Design review of the part built by this model. Coordinates are the model's own, in mm. Face numbers are marked on the shaded views. A direction names the side the tool comes from. Give positions to 0.01 mm unless a question says otherwise; leave off trailing zeros. Order: outer loops, then holes, each group sorted by start corner. A loop starts at its lowest first (then second) coordinate and runs counter-clockwise, first axis right, second up. Notation, with made-up numbers: M -4,42 L 7,42 A6 cw 7,49 Z; hole C 25,21 d8. An arc over 180 degrees is marked long. Answer as a JSON object with one key per item and string values.
from build123d import *

# Parameters (mm, degrees)
SKETCH1_R               = 19
SKETCH1_R_2             = 10
BOSS_EXTRUDE1_DEPTH     = 1.5
SKETCH2_R               = 1.55
CUT_EXTRUDE1_DEPTH      = 27.911893282
SKETCH3_R               = 10.5
BOSS_EXTRUDE2_DEPTH     = 3
CHAMFER2_SIZE           = 0.4
SKETCH4_R               = 5
BOSS_EXTRUDE3_DEPTH     = 3
CUT_EXTRUDE2_DEPTH      = 27.147397772
CUT_EXTRUDE2_DEPTH_BACK = 27.147397772
SKETCH4_3_R             = 2.5


with BuildPart() as part:
    # Sketch1 → Boss-Extrude1 (new body)
    with BuildSketch(Plane(origin=(0, 0, 0), x_dir=(1, 0, 0), z_dir=(0, 1, 0))):
        with Locations(Location((0, 0, 0), (0, 0, 270))):
            Circle(SKETCH1_R)
        with Locations(Location((0, 0, 0), (0, 0, 270))):
            Circle(SKETCH1_R_2, mode=Mode.SUBTRACT)
    extrude(amount=BOSS_EXTRUDE1_DEPTH)

    # Sketch2 → Cut-Extrude1 (cut, through all)
    with BuildSketch(Plane(origin=(0, 1.5, 0), x_dir=(1, 0, 0), z_dir=(0, 1, 0))):
        with Locations(Location((-8.485, 12.005347771, 0), (0, 0, 270))):
            Circle(SKETCH2_R)
        with Locations(Location((6.154436151, 13.350899437, 0), (0, 0, 270))):
            Circle(SKETCH2_R)
        with Locations(Location((14.639436151, 1.345551666, 0), (0, 0, 270))):
            Circle(SKETCH2_R)
        with Locations(Location((8.485, -12.005347771, 0), (0, 0, 270))):
            Circle(SKETCH2_R)
        with Locations(Location((-6.154436151, -13.350899437, 0), (0, 0, 270))):
            Circle(SKETCH2_R)
        with Locations(Location((-14.639436151, -1.345551666, 0), (0, 0, 270))):
            Circle(SKETCH2_R)
        Polygon((-9.483235294, 16.464150399), (6.878487463, 17.711194489), (6.645170501, 20.772407387), (-9.483235294, 19.543146054), align=None)
        Polygon((9.483235294, -16.464150399), (9.716552256, -19.525363297), (-6.411853538, -20.75462463), (-6.878487463, -17.711194489), align=None)
    extrude(amount=-CUT_EXTRUDE1_DEPTH, mode=Mode.SUBTRACT)

    # Sketch3 → Boss-Extrude2 (add)
    with BuildSketch(Plane(origin=(0, 1.5, 0), x_dir=(1, 0, 0), z_dir=(0, 1, 0))):
        with Locations(Location((0, 0, 0), (0, 0, 270))):
            Circle(SKETCH3_R)
    extrude(amount=BOSS_EXTRUDE2_DEPTH)

    # Chamfer2
    chamfer2_edges = [part.edges().sort_by_distance(p)[0] for p in [
        (-18.945053245, 0, 1.443938211),
        (18.945053245, 0, -1.443938211),
        (-1.302373916, 0, -17.087672444),
        (1.302373916, 0, 17.087672444),
    ]]
    chamfer(chamfer2_edges, length=CHAMFER2_SIZE)

    # Sketch4 → Boss-Extrude3 (add)
    with BuildSketch(Plane.XZ.offset(-1.5)):
        with Locations(Location((0, 0, 0), (0, 0, 90))):
            Circle(SKETCH4_R)
    extrude(amount=BOSS_EXTRUDE3_DEPTH)

    # Sketch4_3 → Cut-Extrude2 (cut, two sides: drawn at the far end of the back side and taken through both)
    with BuildSketch(Plane.XZ.offset(-1.5).offset(-CUT_EXTRUDE2_DEPTH_BACK)):
        with Locations(Location((0, 0, 0), (0, 0, 270))):
            Circle(SKETCH4_3_R)
    extrude(amount=CUT_EXTRUDE2_DEPTH + CUT_EXTRUDE2_DEPTH_BACK, mode=Mode.SUBTRACT)


solid = part.part
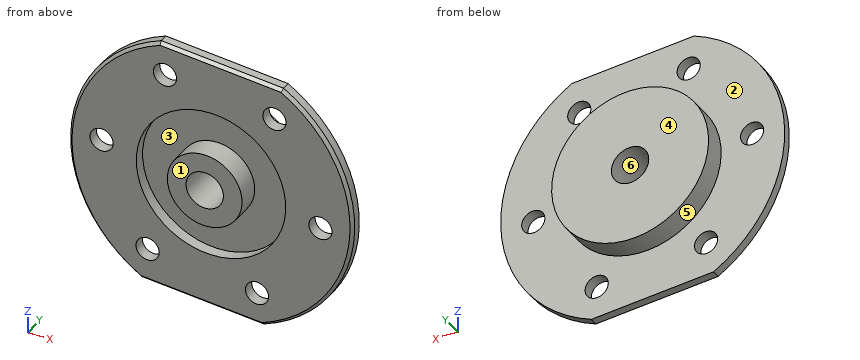
(1) To check wall thickness, follow L1, parallel to X at y = 0.95, z = 4; L2, parallel to X at y = 0.55, z = 0; L3, parallel to Y at x = -12.5, z = 0.5. State the ranges of each line that lie inside material, in increasing order. Write a range as from..to.
Checked values:
{"L1": "x = -18.57..-9.17, -3..3, 9.17..18.57", "L2": "x = -19..-15.41, -13.87..-10, -5..-2.5, 2.5..5, 10..13.87, 15.41..19", "L3": "y = 0..1.5"}
(2) We need section B-B (y = 1.95). Write out the cut boundary in (x, z).
Checked values:
{"outline": "C 0,0 d21; hole C 0,0 d5"}
(3) We need section C-C (z = -12.5). Count the separate pieces of the cut face and the enclosed holes in it, plus the area to 3 significant figures.
Checked values:
{"separate pieces": "3", "enclosed holes": "0", "area": "34.4 mm^2"}
(4) Tool access review of the marked faces 1, 2 and 3: name each direction out of +Z, -Z, +X, -X, +Y, -Y from which nothing blocks a thin tool from reaching the whole face with its end or side.
Checked values:
{"face 1": "+Z, -Z, +X, -X, -Y", "face 2": "+Y", "face 3": "-Y"}
(5) We need section A-A (x = 0). Write out the cut boundary in (y, z), plus the area to 3 significant figures.
Checked values:
{"outline": "M -1.5,-5 L 1.5,-5 L 1.5,-10 L 0,-10 L 0,-16.79 L 0.4,-17.19 L 1.5,-17.19 L 1.5,-10.5 L 4.5,-10.5 L 4.5,-2.5 L -1.5,-2.5 Z; M -1.5,2.5 L 4.5,2.5 L 4.5,10.5 L 1.5,10.5 L 1.5,17.19 L 0.4,17.19 L 0,16.79 L 0,10 L 1.5,10 L 1.5,5 L -1.5,5 Z", "area": "84.4 mm^2"}
(6) Draft analysis for pull direction X (two halves, no side actions). For the marked faces 4, 5 and 6, state which applies: +X half, -X half, draft (parallel to the pull), parting line (faces both ways), or undercut.
Checked values:
{"face 4": "draft", "face 5": "parting line", "face 6": "undercut"}
(7) Insertion check: pin 1 (5 mm diameter, centred on x = -6.15, z = 13.35, fed in from -Y); pin 2 (2 mm diameter, centred on x = -14.5, z = 3.5, fed in from +Y). Each pin has a flat end and moves straight along its axis. Give the tip position at first contact, or say it passes through.
Checked values:
{"pin 1": "stops at y = 0", "pin 2": "stops at y = 1.5"}
